Read the model definition and answer for the solid it produces. Units are mm, in the model's axes. Round coordinates to 2 decimals unless told otherwise and drop trailing zeros. Order: outer loops, then holes, each group sorted by start corner. A loop starts at its lowest first (then second) coordinate and runs counter-clockwise, first axis right, second up.
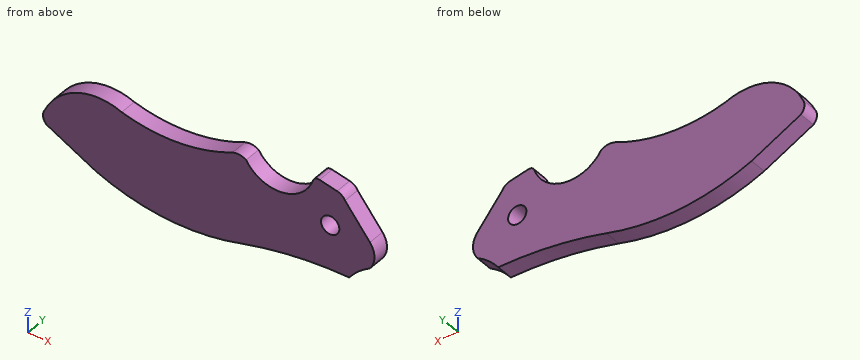
from build123d import *

# Parameters (mm, degrees)
F0_R     = 3.32764
F1_DEPTH = 6.35


with BuildPart() as f1:
    # F0 (on Front) → F1 (new body)
    with BuildSketch(Plane.XZ):
        with BuildLine():
            ThreePointArc((10.863197, -3.101384), (-9.116668, -7.905005), (-29.521924, -5.476979))
            ThreePointArc((-29.521924, -5.476979), (-45.742293, -5.257841), (-57.473989, -16.46122))
            ThreePointArc((-57.473989, -16.46122), (-58.148469, -19.15893), (-56.883303, -21.635201))
            ThreePointArc((-56.883303, -21.635201), (-47.926878, -26.330705), (-38.960246, -31.006687))
            ThreePointArc((-38.960246, -31.006687), (-12.808025, -37.551213), (14.029663, -35.000129))
            ThreePointArc((14.029663, -35.000129), (33.535174, -31.476841), (53.343166, -30.754377))
            ThreePointArc((53.343166, -30.754377), (56.744891, -27.089985), (60.856728, -24.245292))
            ThreePointArc((60.856728, -24.245292), (62.508975, -19.496347), (60.856728, -14.747403))
            Line((60.856728, -14.747403), (51.819268, -3.331661))
            ThreePointArc((51.819268, -3.331661), (50.614082, -1.893648), (48.914772, -1.098222))
            Line((48.914772, -1.098222), (42.531531, 0.329607))
            ThreePointArc((42.531531, 0.329607), (41.058171, 0.198446), (40.120659, -0.945698))
            ThreePointArc((40.120659, -0.945698), (28.833955, -10.074921), (15.773744, -3.73747))
            ThreePointArc((15.773744, -3.73747), (13.389868, -2.868245), (10.863197, -3.101384))
        make_face()
        with Locations((46.395506, -14.617501)):
            Circle(F0_R, mode=Mode.SUBTRACT)
    extrude(amount=F1_DEPTH)


solid = f1.part
Q1. Straight lines are drawn through the part: probe 1 along Z at (x, y) = (46, -1.25); probe 2 along Z at (x, y) = (45, -1); probe 3 along X at (y, z) = (-4, -15.5). For each, find the intervals that lie inside material, in ascending order.
Outcome:
probe 1: z = -30.69 to -17.92, -11.31 to -0.45
probe 2: z = -30.71 to -17.64, -11.6 to -0.22
probe 3: x = -57.02 to 43.19, 49.6 to 61.38
Q2. A cutting plane is placed at A-A, the plane x = 45. Give the vertices of the cut face in (y, z), plus the area to 3 significant figures.
Outcome:
outline: (-6.35, -30.71) - (0, -30.71) - (0, -17.64) - (-6.35, -17.64) - close; (-6.35, -11.6) - (0, -11.6) - (0, -0.22) - (-6.35, -0.22) - close
area: 155 mm2
Q3. A cutting plane is placed at D-D, the plane x = -16.5. Give the vertices of the cut face in (y, z).
Outcome:
outline: (-6.35, -37.19) - (0, -37.19) - (0, -7.87) - (-6.35, -7.87) - close
Q4. A cutting plane is placed at C-C, the plane x = 26.5. Give the vertices of the cut face in (y, z).
Outcome:
outline: (-6.35, -32.42) - (0, -32.42) - (0, -10.14) - (-6.35, -10.14) - close
Q5. A cutting plane is placed at B-B, the plane y = -3.5. Give the vertices of the cut face in (x, z), plus the area to 3 significant figures.
Outcome:
outline: (-57.47, -16.46) arc R3.96 ccw to (-56.88, -21.64) arc R4642.23 ccw to (-38.96, -31.01) arc R79.68 ccw to (14.03, -35) arc R139.46 cw to (53.34, -30.75) arc R23.05 cw to (60.86, -24.25) arc R7.65 ccw to (60.86, -14.75) - (51.82, -3.33) arc R4.34 ccw to (48.91, -1.1) - (42.53, 0.33) arc R1.91 ccw to (40.12, -0.95) arc R13.54 cw to (15.77, -3.74) arc R5.79 ccw to (10.86, -3.1) arc R58.29 cw to (-29.52, -5.48) arc R21.44 ccw to start; hole circle Ø6.66 at (46.4, -14.62)
area: 3,080 mm2
Q6. A flat-ended cylindrical pin translates along its axis: pin 1 (2 mm diameter, centred on y = -5.5, z = -22, fed in from +X). Find the tip coordinate at first contact, or state that the pin passes through.
Outcome:
pin 1: stops at x = 62.36
